Read the model definition and answer for the solid it produces. Units are mm, in the model's axes. Give positions to 0.01 mm unless a question says otherwise; leave off trailing zeros. Loops run counter-clockwise (first coordinate to the right, second up) from the corner with the lowest first, then second, coordinate; pieces in that order, holes last. Notation, with made-up numbers: (59, 84) -> (111, 84) arc R23 cw to (111, 115) -> close; hole circle Ø10 at (-25, 18). An arc over 180 degrees is marked (long way). Return JSON: item names as keys, results as strings. Group by question number.
from build123d import *

# Parameters (mm, degrees)
SKETCH_1_W          = 41
SKETCH_1_H          = 40
SKETCH_1_R          = 1.25
SKETCH_1_R_2        = 1
EXTRUDE_1_DEPTH     = 2
SKETCH_4_W          = 18
SKETCH_4_H          = 22
CUT_EXTRUDE_1_DEPTH = 2
FILLET_2_R          = 2.5
FILLET_3_R          = 5
CUT_EXTRUDE_2_DEPTH = 2
FILLET_4_R          = 1
SKETCH_6_W          = 18
SKETCH_6_H          = 14
CUT_EXTRUDE_3_DEPTH = 10
FILLET_5_R          = 1
SKETCH_7_R          = 1
CUT_EXTRUDE_4_DEPTH = 10


with BuildPart() as part:
    # 草圖1 → 填料-伸長1 (new body)
    with BuildSketch(Plane.XY):
        with Locations((-5.216213198, -9.8375)):
            Rectangle(SKETCH_1_W, SKETCH_1_H)
        with Locations((-17.216213198, 3.6625)):
            Circle(SKETCH_1_R, mode=Mode.SUBTRACT)
        with Locations((-17.216213198, -23.3375)):
            Circle(SKETCH_1_R, mode=Mode.SUBTRACT)
        with Locations((12.783786802, -23.3375)):
            Circle(SKETCH_1_R, mode=Mode.SUBTRACT)
        with Locations((12.783786802, 3.6625)):
            Circle(SKETCH_1_R, mode=Mode.SUBTRACT)
        with Locations((-23.716213198, -9.8375)):
            Circle(SKETCH_1_R_2, mode=Mode.SUBTRACT)
    extrude(amount=EXTRUDE_1_DEPTH)

    # 草圖4 → 除料-伸長1 (cut)
    with BuildSketch(Plane(origin=(0, 0, 0), x_dir=(-1, 0, 0), z_dir=(0, 0, -1))):
        with Locations((-6.283786802, -9.8375)):
            Rectangle(SKETCH_4_W, SKETCH_4_H)
    extrude(amount=-CUT_EXTRUDE_1_DEPTH, mode=Mode.SUBTRACT)

    # 圓角2
    fillet_2_edges = [part.edges().sort_by_distance(p)[0] for p in [
        (15.283786802, -20.8375, 1),
        (15.283786802, 1.1625, 1),
    ]]
    fillet(fillet_2_edges, radius=FILLET_2_R)

    # 圓角3
    fillet_3_edges = [part.edges().sort_by_distance(p)[0] for p in [
        (-2.716213198, 1.1625, 1),
        (-2.716213198, -20.8375, 1),
    ]]
    fillet(fillet_3_edges, radius=FILLET_3_R)

    # 草圖5 → 除料-伸長2 (cut)
    with BuildSketch(Plane(origin=(0, 0, 0), x_dir=(-1, 0, 0), z_dir=(0, 0, -1))):
        with BuildLine():
            Line((7.716213198, -3.8375), (7.716213198, -15.8375))
            ThreePointArc((7.716213198, -15.8375), (9.180679292, -19.373033906), (12.716213198, -20.8375))
            Line((12.716213198, -20.8375), (16.216213198, -20.8375))
            ThreePointArc((16.216213198, -20.8375), (19.751747104, -19.373033906), (21.216213198, -15.8375))
            Line((21.216213198, -15.8375), (21.216213198, -3.8375))
            ThreePointArc((21.216213198, -3.8375), (19.751747104, -0.301966094), (16.216213198, 1.1625))
            Line((16.216213198, 1.1625), (12.716213198, 1.1625))
            ThreePointArc((12.716213198, 1.1625), (9.204017559, -0.325304361), (7.716213198, -3.8375))
        make_face()
    extrude(amount=-CUT_EXTRUDE_2_DEPTH, mode=Mode.SUBTRACT)

    # 圓角4
    fillet_4_edges = [part.edges().sort_by_distance(p)[0] for p in [
        (-25.716213198, 10.1625, 1),
        (15.283786802, 10.1625, 1),
        (15.283786802, -29.8375, 1),
        (-25.716213198, -29.8375, 1),
    ]]
    fillet(fillet_4_edges, radius=FILLET_4_R)

    # 草圖6 → 除料-伸長3 (cut)
    with BuildSketch(Plane(origin=(0, 0, 0), x_dir=(-1, 0, 0), z_dir=(0, 0, -1))):
        with Locations((-6.283786802, 3.1625)):
            Rectangle(SKETCH_6_W, SKETCH_6_H)
        with Locations((-6.283786802, -22.8375)):
            Rectangle(SKETCH_6_W, SKETCH_6_H)
    extrude(amount=-CUT_EXTRUDE_3_DEPTH, mode=Mode.SUBTRACT)

    # 圓角5
    fillet_5_edges = [part.edges().sort_by_distance(p)[0] for p in [
        (-2.716213198, 10.1625, 1),
        (-2.716213198, -29.8375, 1),
    ]]
    fillet(fillet_5_edges, radius=FILLET_5_R)

    # 草圖7 → 除料-伸長4 (cut)
    with BuildSketch(Plane(origin=(0, 0, 0), x_dir=(-1, 0, 0), z_dir=(0, 0, -1))):
        with Locations((4.716213198, -27.8375)):
            Circle(SKETCH_7_R)
        with Locations((12.716213198, -27.8375)):
            Circle(SKETCH_7_R)
        with Locations(Location((12.716213198, 8.1625, 0), (0, 0, 180))):
            Circle(SKETCH_7_R)
        with Locations(Location((4.716213198, 8.1625, 0), (0, 0, 180))):
            Circle(SKETCH_7_R)
    extrude(amount=-CUT_EXTRUDE_4_DEPTH, mode=Mode.SUBTRACT)


solid = part.part
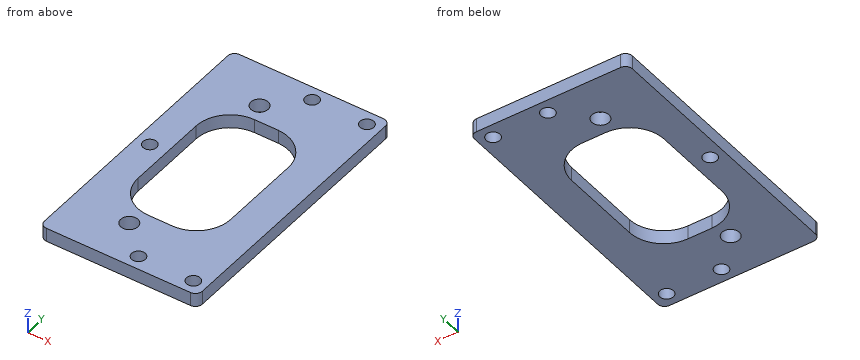
1. Section A-A on y = -12 is taken. Determine the outline of the cut face in (x, z), then the cut area to 3 significant figures.
2. A flat-ended cylindrical pin translates along its axis: pin 1 Ø8 at (x, y) = (-16.5, 3) entering from +Z. Find the tip coordinate at first contact, or state that the pin passes through.
3. Section D-D on x = -4.5 is taken. Determine the outline of the cut face in (y, z), then the cut area to 3 significant figures.
4. Section C-C on z = 1.45 is taken. State how many separate pieces and enclosed holes the cut face has, then the cut area to 3 significant figures.
5. Straight lines are drawn through the part: line 1 (X direction, y = -6, z = 0.5); line 2 (Y direction, x = -4.25, z = 0.3); line 3 (X direction, y = -10, z = 0.9). For each, find the intervals that lie inside material, in ascending order. Write a range as from..to.
6. Section B-B on x = -15.5 is taken. Determine the outline of the cut face in (y, z).
Completed:
{
 "1": {"outline": "(-25.72, 0) -> (-21.22, 0) -> (-21.22, 2) -> (-25.72, 2) -> close; (-7.72, 0) -> (-2.72, 0) -> (-2.72, 2) -> (-7.72, 2) -> close", "area": "19.0 mm²"},
 "2": {"pin 1": "stops at z = 2"},
 "3": {"outline": "(-29.84, 0) -> (-28.81, 0) -> (-28.81, 2) -> (-29.84, 2) -> close; (-26.86, 0) -> (7.19, 0) -> (7.19, 2) -> (-26.86, 2) -> close; (9.14, 0) -> (10.16, 0) -> (10.16, 2) -> (9.14, 2) -> close", "area": "72.2 mm²"},
 "4": {"separate pieces": "1", "enclosed holes": "8", "area": "618 mm²"},
 "5": {"line 1": "x = -25.72..-21.22, -7.72..-2.72", "line 2": "y = -29.84..-28.72, -26.95..7.28, 9.05..10.16", "line 3": "x = -25.72..-24.7, -22.73..-21.22, -7.72..-2.72"},
 "6": {"outline": "(-29.84, 0) -> (-20.84, 0) -> (-20.84, 2) -> (-29.84, 2) -> close; (1.16, 0) -> (10.16, 0) -> (10.16, 2) -> (1.16, 2) -> close"}
}
